Design review of the part shown in the three views and the two pictorial views. Dimensions are in mm from the part's minimum x, y and z. Give positions to 0.01 mm unless a question says otherwise; leave off trailing zeros. Order: outer loops, then holes, each group sorted by start corner. A loop starts at its lowest first (then second) coordinate and runs counter-clockwise, first axis right, second up.
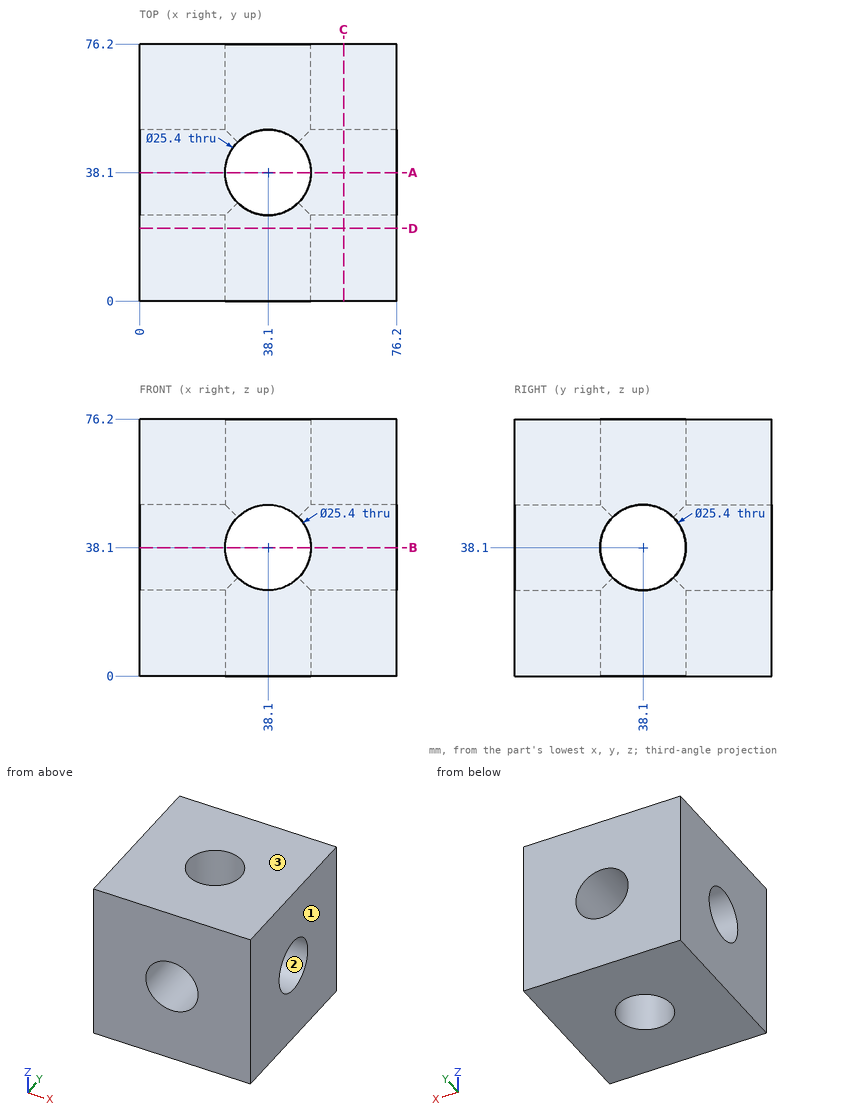
Item 1: Take a section at C-C (x = 60.5). Give the boundary of the cut face in (y, z).
Values found:
outline: (0, 0) - (76.2, 0) - (76.2, 76.2) - (0, 76.2) - close; hole circle Ø25.4 at (38.1, 38.1)
Item 2: For line 1 (X direction, y = 63, z = 38), list the stretches that pass through material, from the lowest coordinate up.
Values found:
line 1: x = 0 to 25.4, 50.8 to 76.2
Item 3: Take a section at A-A (y = 38.1). Give the boundary of the cut face in (x, z).
Values found:
outline: (0, 0) - (25.4, 0) - (25.4, 25.4) - (0, 25.4) - close; (0, 50.8) - (25.4, 50.8) - (25.4, 76.2) - (0, 76.2) - close; (50.8, 0) - (76.2, 0) - (76.2, 25.4) - (50.8, 25.4) - close; (50.8, 50.8) - (76.2, 50.8) - (76.2, 76.2) - (50.8, 76.2) - close
Item 4: Draft analysis for pull direction Z (two halves, no side actions). For the marked faces 1, 2 and 3, state which applies: released by +Z, released by -Z, zero draft, split by the parting line, or undercut.
Values found:
face 1: zero draft
face 2: undercut
face 3: released by +Z
